```python
from build123d import *

# Parameters (mm, degrees)
SKETCH1_W           = 22
SKETCH1_H           = 20
SKETCH1_R           = 0.511248757
BOSS_EXTRUDE1_DEPTH = 12
SKETCH1_3_R         = 1.525
SKETCH1_3_R_2       = 1.6
SKETCH1_3_R_3       = 1.55
SKETCH1_3_R_4       = 1.625
SKETCH1_3_R_5       = 1.65
SKETCH1_3_R_6       = 1.575
CUT_EXTRUDE1_DEPTH  = 20.104973175
CHAMFER1_SIZE       = 0.5


with BuildPart() as part:
    # Sketch1 → Boss-Extrude1 (new body)
    with BuildSketch(Plane(origin=(0, 0, 0), x_dir=(1, 0, 0), z_dir=(0, 1, 0))):
        Rectangle(SKETCH1_W, SKETCH1_H)
        with Locations(Location((-9.381564608, 8.528695098, 0), (0, 0, 270))):
            Circle(SKETCH1_R, mode=Mode.SUBTRACT)
    extrude(amount=-BOSS_EXTRUDE1_DEPTH)

    # Sketch1_3 → Cut-Extrude1 (cut, through all)
    with BuildSketch(Plane(origin=(0, 0, 0), x_dir=(1, 0, 0), z_dir=(0, 1, 0))):
        with Locations(Location((-6, 5, 0), (0, 0, 270))):
            Circle(SKETCH1_3_R)
        with Locations(Location((-6, -5, 0), (0, 0, 270))):
            Circle(SKETCH1_3_R_2)
        with Locations(Location((0, 5, 0), (0, 0, 270))):
            Circle(SKETCH1_3_R_3)
        with Locations(Location((0, -5, 0), (0, 0, 270))):
            Circle(SKETCH1_3_R_4)
        with Locations(Location((6, -5, 0), (0, 0, 270))):
            Circle(SKETCH1_3_R_5)
        with Locations(Location((6, 5, 0), (0, 0, 270))):
            Circle(SKETCH1_3_R_6)
    extrude(amount=-CUT_EXTRUDE1_DEPTH, mode=Mode.SUBTRACT)

    # Chamfer1
    chamfer1_edges = [part.edges().sort_by_distance(p)[0] for p in [
        (6, 0, 3.35),
        (0, 0, 3.375),
        (0, 0, -6.55),
        (-6, 0, 3.4),
        (6, 0, -6.575),
        (-6, 0, -6.525),
    ]]
    chamfer(chamfer1_edges, length=CHAMFER1_SIZE)


solid = part.part
```
Check sheet for the modelled part. Datum: model origin and axes. Units: mm. Round coordinates to 2 decimals unless told otherwise and drop trailing zeros. Loops run counter-clockwise (first coordinate to the right, second up) from the corner with the lowest first, then second, coordinate; pieces in that order, holes last. Notation, with made-up numbers: (70.5, 2.25) - (79.5, 2.25) arc R26 cw to (79.5, 29.25) - close; hole circle Ø5 at (-37.5, 33.5). An arc over 180 degrees is marked (long way). Write item = value, one per line. Start each with the question number.
Q1. Release check for a two-part mould opening along X. For faces 1 (the face through (-11, -6, 0)), 2 (the face through (5, -6.17, 3.69)), 3 (the face through (0, 0, 0)) record: pulls with the +X half, pulls with the -X half, needs draft (parallel to the pull), parting line crosses it, or undercut.
Q2. Section check B-B (x = -6). Record the boundary of the cut face in (y, z) (3 decimals).
Q3. Thickness scan on L1, parallel to X at y = -8, z = -5 (3 decimals); L2, parallel to X at y = -5.5, z = 5 (3 decimals); L3, parallel to Z at x = -5, y = -10.5. Record the ranges inside material, lowest first.
Q4. Section check C-C (y = -3.25). Count the separate pieces of the cut face and the enclosed holes in it, plus the area to 3 significant figures.
Q5. Depth check by flat-ended pin: P1, Ø0.9, axis at x = -9.38, z = -8.53, coming from the +Y side. Enter the tip coordinate at first touch or a pass-through.
Q6. Section check A-A (z = -5). Record the boundary of the cut face in (x, y) (3 decimals).
Q7. Section check D-D (z = 5). Record the boundary of the cut face in (x, y) (3 decimals).
Derived:
q1.face_1 = pulls with the -X half
q1.face_2 = undercut
q1.face_3 = needs draft
q2.outline = (-12, -10) - (0, -10) - (0, -7.025) - (-0.5, -6.525) - (-12, -6.525) - close; (-12, -3.475) - (-0.5, -3.475) - (0, -2.975) - (0, 2.9) - (-0.5, 3.4) - (-12, 3.4) - close; (-12, 6.6) - (-0.5, 6.6) - (0, 7.1) - (0, 10) - (-12, 10) - close
q3.L1 = -11 to -7.525, -4.475 to -1.55, 1.55 to 4.425, 7.575 to 11
q3.L2 = -11 to -7.6, -4.4 to -1.625, 1.625 to 4.35, 7.65 to 11
q3.L3 = -10 to -6.15, -3.85 to 3.75, 6.25 to 10
q4.separate_pieces = 1
q4.enclosed_holes = 7
q4.area = 392 mm^2
q5.P1 = through
q6.outline = (-11, -12) - (-7.525, -12) - (-7.525, -0.5) - (-8.025, 0) - (-11, 0) - close; (-4.475, -12) - (-1.55, -12) - (-1.55, -0.5) - (-2.05, 0) - (-3.975, 0) - (-4.475, -0.5) - close; (1.55, -12) - (4.425, -12) - (4.425, -0.5) - (3.925, 0) - (2.05, 0) - (1.55, -0.5) - close; (7.575, -12) - (11, -12) - (11, 0) - (8.075, 0) - (7.575, -0.5) - close
q7.outline = (-11, -12) - (-7.6, -12) - (-7.6, -0.5) - (-8.1, 0) - (-11, 0) - close; (-4.4, -12) - (-1.625, -12) - (-1.625, -0.5) - (-2.125, 0) - (-3.9, 0) - (-4.4, -0.5) - close; (1.625, -12) - (4.35, -12) - (4.35, -0.5) - (3.85, 0) - (2.125, 0) - (1.625, -0.5) - close; (7.65, -12) - (11, -12) - (11, 0) - (8.15, 0) - (7.65, -0.5) - close
